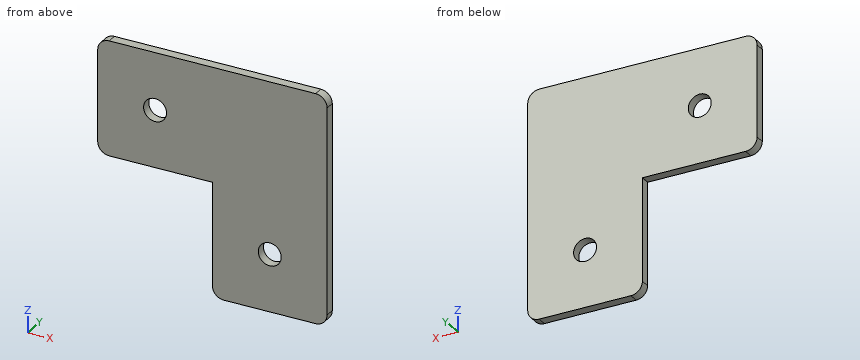
```python
from build123d import *

# Parameters (mm, degrees)
BOSS_EXTRUDE1_DEPTH = 2.5
FILLET1_R           = 3
FILLET2_R           = 3
FILLET3_R           = 3
FILLET4_R           = 3
FILLET5_R           = 3
SKETCH2_R           = 3
CUT_EXTRUDE1_DEPTH  = 3


with BuildPart() as part:
    # Sketch1 → Boss-Extrude1 (new body)
    with BuildSketch(Plane(origin=(0, 0, 0), x_dir=(1, 0, 0), z_dir=(0, 1, 0))):
        Polygon((-12.469879518, 24.84939759), (17.530120482, 24.84939759), (17.530120482, -35.15060241), (-12.469879518, -35.15060241), (-42.469879518, -35.15060241), (-42.469879518, -5.15060241), (-12.469879518, -5.15060241), align=None)
    extrude(amount=BOSS_EXTRUDE1_DEPTH)

    # Fillet1
    fillet1_edges = [part.edges().sort_by_distance(p)[0] for p in [
        (-42.469879518, 1.25, 5.15060241),
    ]]
    fillet(fillet1_edges, radius=FILLET1_R)

    # Fillet2
    fillet2_edges = [part.edges().sort_by_distance(p)[0] for p in [
        (-42.469879518, 1.25, 35.15060241),
    ]]
    fillet(fillet2_edges, radius=FILLET2_R)

    # Fillet3
    fillet3_edges = [part.edges().sort_by_distance(p)[0] for p in [
        (17.530120482, 1.25, 35.15060241),
    ]]
    fillet(fillet3_edges, radius=FILLET3_R)

    # Fillet4
    fillet4_edges = [part.edges().sort_by_distance(p)[0] for p in [
        (17.530120482, 1.25, -24.84939759),
    ]]
    fillet(fillet4_edges, radius=FILLET4_R)

    # Fillet5
    fillet5_edges = [part.edges().sort_by_distance(p)[0] for p in [
        (-12.469879518, 1.25, -24.84939759),
    ]]
    fillet(fillet5_edges, radius=FILLET5_R)

    # Sketch2 → Cut-Extrude1 (cut)
    with BuildSketch(Plane(origin=(0, 2.5, 0), x_dir=(1, 0, 0), z_dir=(0, 1, 0))):
        with Locations((2.530120482, 9.84939759)):
            Circle(SKETCH2_R)
        with Locations((-27.469879518, -20.15060241)):
            Circle(SKETCH2_R)
    extrude(amount=-CUT_EXTRUDE1_DEPTH, mode=Mode.SUBTRACT)


solid = part.part
```
The listing builds one solid part. Answer for the finished solid, in the listing's coordinates (mm). Give positions to 0.01 mm unless a question says otherwise; leave off trailing zeros. Order: outer loops, then holes, each group sorted by start corner. A loop starts at its lowest first (then second) coordinate and runs counter-clockwise, first axis right, second up. Notation, with made-up numbers: (-10, -2) -> (11, -2) arc R16 ccw to (11, 26) -> close; hole circle Ø4 at (39.25, 61). An arc over 180 degrees is marked (long way). Answer as CSV lines item,"result". Start each with the question number.
Q1. Find the intervals of material crossed by L1, parallel to X at y = 1.15, z = 3; L2, parallel to Z at x = -31.5, y = 0.8; L3, parallel to Z at x = -30, y = 1.8, in increasing order.
Q2. Given pin 1 (0.8 mm diameter, centred on x = -32.5, y = 1, fed in from -Z); pin 2 (5.5 mm diameter, centred on x = 2.53, z = -9.85, fed in from -Y), each flat-ended and moving along its own axis, determine where each tip first touches the part or whether it passes through.
Q3. A cutting plane is placed at C-C (x = -26.5). Determine the outline of the cut face in (y, z).
Q4. A cutting plane is placed at A-A (z = -8). Determine the outline of the cut face in (x, y), then the cut area to 3 significant figures.
Q5. A cutting plane is placed at B-B (y = 1.6). Determine the outline of the cut face in (x, z), then the cut area to 3 significant figures.
Q6. A cutting plane is placed at D-D (z = -14). Determine the outline of the cut face in (x, y).
Results found:
1,L1,"-12.47 to 17.53"
1,L2,"5.15 to 35.15"
1,L3,"5.15 to 18.54, 21.76 to 35.15"
2,pin 1,"z = 5.15"
2,pin 2,"through"
3,outline,"(0, 5.15) -> (2.5, 5.15) -> (2.5, 17.31) -> (0, 17.31) -> close; (0, 22.99) -> (2.5, 22.99) -> (2.5, 35.15) -> (0, 35.15) -> close"
4,outline,"(-12.47, 0) -> (0.17, 0) -> (0.17, 2.5) -> (-12.47, 2.5) -> close; (4.89, 0) -> (17.53, 0) -> (17.53, 2.5) -> (4.89, 2.5) -> close"
4,area,"63.2 mm2"
5,outline,"(-42.47, 8.15) arc R3 ccw to (-39.47, 5.15) -> (-12.47, 5.15) -> (-12.47, -21.85) arc R3 ccw to (-9.47, -24.85) -> (14.53, -24.85) arc R3 ccw to (17.53, -21.85) -> (17.53, 32.15) arc R3 ccw to (14.53, 35.15) -> (-39.47, 35.15) arc R3 ccw to (-42.47, 32.15) -> close; hole circle Ø6 at (-27.47, 20.15); hole circle Ø6 at (2.53, -9.85)"
5,area,"2,630 mm2"
6,outline,"(-12.47, 0) -> (17.53, 0) -> (17.53, 2.5) -> (-12.47, 2.5) -> close"
